from build123d import *

# Parameters (mm, degrees)
SKETCH1_W            = 90
SKETCH1_H            = 90
BOSS_EXTRUDE1_DEPTH  = 2.25
SKETCH2_R            = 2.5
CUT_EXTRUDE1_DEPTH   = 0.5
FILLET1_R            = 7
M4_CLEARANCE_HOLE1_D = 4.5


with BuildPart() as part:
    # Sketch1 → Boss-Extrude1 (new body)
    with BuildSketch(Plane(origin=(0, 0, 0), x_dir=(1, 0, 0), z_dir=(0, 1, 0))):
        Rectangle(SKETCH1_W, SKETCH1_H)
    extrude(amount=BOSS_EXTRUDE1_DEPTH)

    # Sketch2 → Cut-Extrude1 (cut)
    with BuildSketch(Plane(origin=(0, 2.25, 0), x_dir=(1, 0, 0), z_dir=(0, 1, 0))):
        with BuildLine():
            ThreePointArc((-35.25, 27), (-32.833630945, 32.833630945), (-27, 35.25))
            Line((-27, 35.25), (27, 35.25))
            ThreePointArc((27, 35.25), (32.833630945, 32.833630945), (35.25, 27))
            Line((35.25, 27), (35.25, -27))
            ThreePointArc((35.25, -27), (32.833630945, -32.833630945), (27, -35.25))
            Line((27, -35.25), (-27, -35.25))
            ThreePointArc((-27, -35.25), (-32.833630945, -32.833630945), (-35.25, -27))
            Line((-35.25, -27), (-35.25, 27))
        make_face()
        with BuildLine():
            Line((-27, -32.25), (27, -32.25))
            ThreePointArc((27, -32.25), (30.712310601, -30.712310601), (32.25, -27))
            Line((32.25, -27), (32.25, 27))
            ThreePointArc((32.25, 27), (30.712310601, 30.712310601), (27, 32.25))
            Line((27, 32.25), (-27, 32.25))
            ThreePointArc((-27, 32.25), (-30.712310601, 30.712310601), (-32.25, 27))
            Line((-32.25, 27), (-32.25, -27))
            ThreePointArc((-32.25, -27), (-30.712310601, -30.712310601), (-27, -32.25))
        make_face(mode=Mode.SUBTRACT)
        with Locations((-20, 20)):
            Circle(SKETCH2_R)
        with Locations((0, 20)):
            Circle(SKETCH2_R)
        with Locations((20, 20)):
            Circle(SKETCH2_R)
        with Locations((20, 0)):
            Circle(SKETCH2_R)
        with Locations((20, -20)):
            Circle(SKETCH2_R)
        with Locations((0, -20)):
            Circle(SKETCH2_R)
        Circle(SKETCH2_R)
        with Locations((-20, 0)):
            Circle(SKETCH2_R)
        with Locations((-20, -20)):
            Circle(SKETCH2_R)
    extrude(amount=-CUT_EXTRUDE1_DEPTH, mode=Mode.SUBTRACT)

    # Fillet1
    fillet1_edges = [part.edges().sort_by_distance(p)[0] for p in [
        (45, 1.125, 45),
        (-45, 1.125, 45),
        (-45, 1.125, -45),
        (45, 1.125, -45),
    ]]
    fillet(fillet1_edges, radius=FILLET1_R)

    # M4 Clearance Hole1 (through all)
    with Locations(Plane(origin=(0, 2.25, 0), x_dir=(1, 0, 0), z_dir=(0, 1, 0))):
        with Locations((-38, 38), (38, 38), (38, -38), (-38, -38)):
            Hole(M4_CLEARANCE_HOLE1_D / 2)


solid = part.part
The listing builds one solid part. Answer for the finished solid, in the listing's coordinates (mm). A direction names the side the tool comes from. Round coordinates to 2 decimals unless told otherwise and drop trailing zeros. Write each loop counter-clockwise with the first axis right and the second up, starting at its lowest first coordinate (ties: lowest second). Pieces come first, ordered by that corner, then holes. Notation, with made-up numbers: M 15.25,-24.75 L 38.25,-24.75 A16 ccw 38.25,-2.75 Z; hole C -8,8 d3. An arc over 180 degrees is marked long. Write each question's results on one line, items separated by ' | '. Start each with the question number.
Item 1: Given pin 1 Ø2 at (x, z) = (7.5, -34.5) entering from +Y; pin 2 Ø1.5 at (x, z) = (20, 19) entering from +Y, each flat-ended and moving along its own axis, determine where each tip first touches the part or whether it passes through.
Item 2: Find section A-A on x = -20. Write down the section's boundary in (y, z), and give its area (3 significant figures).
Item 3: Which of the six approach directions +Z, -Z, +X, -X, +Y, -Y give full straight-line access (tool end or side, diameter ignored) to faces 1 (the flat face through (0, 1.75, 20)), 2 (the flat face through (-1, 1, 45))?
Item 4: Straight lines are drawn through the part: probe 1 along Z at (x, y) = (-12.5, 1.8); probe 2 along Z at (x, y) = (20, 2.1). For each, find the intervals that lie inside material, in ascending order.
Item 5: The mould has two halves that part along Z. Classify faces 3 (the cylindrical face through (17.5, 2, 19.9)), 4 (the cylindrical face through (-43, 1.1, 42.9)), 5 (the flat face through (0, 2.25, -8)): +Z half, -Z half, draft (parallel to the pull), parting line (faces both ways), or undercut.
Answer block:
1) pin 1: stops at y = 2.25 | pin 2: stops at y = 1.75
2) outline: M 0,-45 L 2.25,-45 L 2.25,-35.25 L 1.75,-35.25 L 1.75,-32.25 L 2.25,-32.25 L 2.25,-22.5 L 1.75,-22.5 L 1.75,-17.5 L 2.25,-17.5 L 2.25,-2.5 L 1.75,-2.5 L 1.75,2.5 L 2.25,2.5 L 2.25,17.5 L 1.75,17.5 L 1.75,22.5 L 2.25,22.5 L 2.25,32.25 L 1.75,32.25 L 1.75,35.25 L 2.25,35.25 L 2.25,45 L 0,45 Z | area: 192 mm²
3) face 1: +Y | face 2: +Z, +X, -X, +Y, -Y
4) probe 1: z = -45 to -35.25, -32.25 to 32.25, 35.25 to 45 | probe 2: z = -45 to -35.25, -32.25 to -22.5, -17.5 to -2.5, 2.5 to 17.5, 22.5 to 32.25, 35.25 to 45
5) face 3: undercut | face 4: +Z half | face 5: draft
